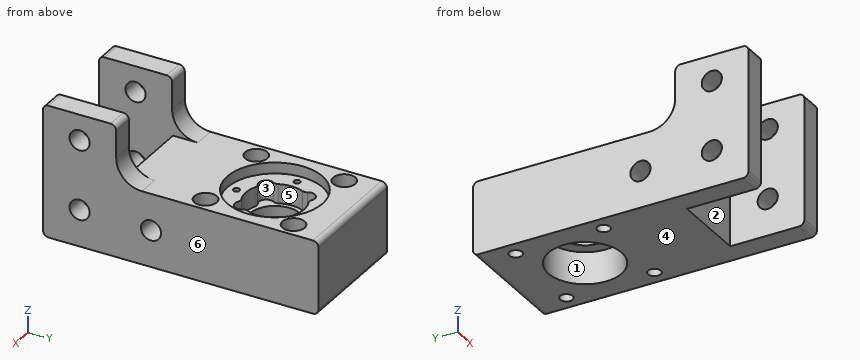
from build123d import *

# Parameters (mm, degrees)
EXTRUDE1_DEPTH      = 10.25
EXTRUDE1_DEPTH_BACK = 10.25
SKETCH1_W           = 20
SKETCH1_H           = 55
EXTRUDE2_DEPTH      = 6
SKETCH4_R           = 2.75
EXTRUDE3_DEPTH      = 78.393878957
SKETCH5_R           = 6.755
EXTRUDE4_DEPTH      = 77.273357078
FILLET2_R           = 1.5
SKETCH_1_W          = 32.5
SKETCH_1_H          = 73.75
CUT_EXTRUDE_1_DEPTH = 77.273357078
FILLET_1_R          = 1.5
SKETCH_2_R          = 13
CUT_EXTRUDE_2_DEPTH = 3
SKETCH_3_R          = 8
SKETCH_3_R_2        = 6.755
CUT_EXTRUDE_3_DEPTH = 5.25
FILLET_2_R          = 1.5
SKETCH_4_R          = 10
CUT_EXTRUDE_4_DEPTH = 8.75
SKETCH_5_R          = 0.875
CUT_EXTRUDE_5_DEPTH = 8
SKETCH_7_R          = 1.75
CUT_EXTRUDE_6_DEPTH = 71.154294238
SKETCH_8_R          = 3.05
CUT_EXTRUDE_7_DEPTH = 5


with BuildPart() as part:
    # Sketch1 → Extrude1 (new, two sides: drawn at the far end of the back side and taken through both)
    with BuildSketch(Plane(origin=(0, 0, 0), x_dir=(0, 0, -1), z_dir=(1, 0, 0)).offset(-EXTRUDE1_DEPTH_BACK)):
        with Locations((0, 37.75)):
            Rectangle(SKETCH1_W, SKETCH1_H)
    extrude(amount=EXTRUDE1_DEPTH + EXTRUDE1_DEPTH_BACK)

    # Sketch2 → Extrude2 (add)
    with BuildSketch(Plane(origin=(10.25, 0, 0), x_dir=(0, 0, -1), z_dir=(1, 0, 0))):
        with BuildLine():
            Line((26, 10), (17, 10))
            ThreePointArc((17, 10), (12.050252532, 12.050252532), (10, 17))
            Line((10, 17), (10, 65.25))
            Line((10, 65.25), (-10, 65.25))
            Line((-10, 65.25), (-10, 17))
            ThreePointArc((-10, 17), (-12.050252532, 12.050252532), (-17, 10))
            Line((-17, 10), (-26, 10))
            Line((-26, 10), (-26, -10))
            Line((-26, -10), (26, -10))
            Line((26, -10), (26, 10))
        make_face()
    extrude2 = extrude(amount=EXTRUDE2_DEPTH)

    # Mirror2: Extrude2 across plane
    add(extrude2.mirror(Plane(origin=(0, 0, 0), x_dir=(0, 0, 1), z_dir=(1, 0, 0))))

    # Sketch4 → Extrude3 (cut, through all)
    with BuildSketch(Plane(origin=(16.25, 0, 0), x_dir=(0, 0, -1), z_dir=(1, 0, 0))):
        Circle(SKETCH4_R)
        with Locations((19, 0)):
            Circle(SKETCH4_R)
        with Locations((-19, 0)):
            Circle(SKETCH4_R)
        with Locations((0, 19.5)):
            Circle(SKETCH4_R)
    extrude(amount=-EXTRUDE3_DEPTH, mode=Mode.SUBTRACT)

    # Sketch5 → Extrude4 (cut, through all)
    with BuildSketch(Plane.XY.offset(10)):
        with Locations((0, 44)):
            Circle(SKETCH5_R)
    extrude(amount=-EXTRUDE4_DEPTH, mode=Mode.SUBTRACT)

    # Fillet2
    fillet2_edges = [part.edges().sort_by_distance(p)[0] for p in [
        (13.25, 10, 26),
        (13.25, -10, 26),
        (13.25, -10, -26),
        (13.25, 10, -26),
        (-13.25, -10, 26),
        (-13.25, 10, 26),
        (-13.25, 10, -26),
        (-13.25, -10, -26),
        (0, 65.25, 10),
        (0, 65.25, -10),
    ]]
    fillet(fillet2_edges, radius=FILLET2_R)

    # Эскиз1 → Вырез-Вытянуть1 (cut, through all)
    with BuildSketch(Plane(origin=(0, 0, -10), x_dir=(-1, 0, 0), z_dir=(0, 0, -1))):
        with Locations((0, 26.875)):
            Rectangle(SKETCH_1_W, SKETCH_1_H)
    extrude(amount=CUT_EXTRUDE_1_DEPTH, mode=Mode.SUBTRACT)

    # Скругление1
    fillet_1_edges = [part.edges().sort_by_distance(p)[0] for p in [
        (-13.25, -10, -10),
        (13.25, -10, -10),
    ]]
    fillet(fillet_1_edges, radius=FILLET_1_R)

    # Эскиз2 → Вырез-Вытянуть2 (cut)
    with BuildSketch(Plane.XY.offset(10)):
        with Locations((0, 44)):
            Circle(SKETCH_2_R)
    extrude(amount=-CUT_EXTRUDE_2_DEPTH, mode=Mode.SUBTRACT)

    # Эскиз3 → Вырез-Вытянуть3 (cut)
    # profile 1 of 5: a face of its own
    with BuildSketch(Plane.XY.offset(7)):
        with Locations((0, 44)):
            Circle(SKETCH_3_R)
        with Locations((0, 44)):
            Circle(SKETCH_3_R_2, mode=Mode.SUBTRACT)
    # profile 2 of 5: a face of its own
    with BuildSketch(Plane.XY.offset(7)):
        with BuildLine():
            ThreePointArc((-6.883199074, 48.076956034), (-5.656854249, 49.656854249), (-4.076956034, 50.883199074))
            ThreePointArc((-4.076956034, 50.883199074), (-7.071067812, 51.071067812), (-6.883199074, 48.076956034))
        make_face()
    # profile 3 of 5: a face of its own
    with BuildSketch(Plane.XY.offset(7)):
        with BuildLine():
            ThreePointArc((4.076956034, 50.883199074), (5.656854249, 49.656854249), (6.883199074, 48.076956034))
            ThreePointArc((6.883199074, 48.076956034), (7.071067812, 51.071067812), (4.076956034, 50.883199074))
        make_face()
    # profile 4 of 5: a face of its own
    with BuildSketch(Plane.XY.offset(7)):
        with BuildLine():
            ThreePointArc((4.076956034, 37.116800926), (7.071067812, 36.928932188), (6.883199074, 39.923043966))
            ThreePointArc((6.883199074, 39.923043966), (5.656854249, 38.343145751), (4.076956034, 37.116800926))
        make_face()
    # profile 5 of 5: a face of its own
    with BuildSketch(Plane.XY.offset(7)):
        with BuildLine():
            ThreePointArc((-6.883199074, 39.923043966), (-7.071067812, 36.928932188), (-4.076956034, 37.116800926))
            ThreePointArc((-4.076956034, 37.116800926), (-5.656854249, 38.343145751), (-6.883199074, 39.923043966))
        make_face()
    extrude(amount=-CUT_EXTRUDE_3_DEPTH, mode=Mode.SUBTRACT)

    # Скругление2
    fillet_2_edges = [part.edges().sort_by_distance(p)[0] for p in [
        (6.883199074, 48.076956034, 4.375),
        (6.883199074, 39.923043966, 4.375),
        (4.076956034, 37.116800926, 4.375),
        (-4.076956034, 37.116800926, 4.375),
        (-6.883199074, 39.923043966, 4.375),
        (-6.883199074, 48.076956034, 4.375),
        (-4.076956034, 50.883199074, 4.375),
        (4.076956034, 50.883199074, 4.375),
    ]]
    fillet(fillet_2_edges, radius=FILLET_2_R)

    # Эскиз4 → Вырез-Вытянуть4 (cut)
    with BuildSketch(Plane(origin=(0, 0, -10), x_dir=(-1, 0, 0), z_dir=(0, 0, -1))):
        with Locations(Location((0, 44, 0), (0, 0, 90))):
            Circle(SKETCH_4_R)
    extrude(amount=-CUT_EXTRUDE_4_DEPTH, mode=Mode.SUBTRACT)

    # Эскиз5 → Вырез-Вытянуть5 (cut)
    with BuildSketch(Plane.XY.offset(7)):
        with Locations((0, 54.5)):
            Circle(SKETCH_5_R)
        with Locations((10.5, 44)):
            Circle(SKETCH_5_R)
        with Locations((0, 33.5)):
            Circle(SKETCH_5_R)
        with Locations((-10.5, 44)):
            Circle(SKETCH_5_R)
    extrude(amount=-CUT_EXTRUDE_5_DEPTH, mode=Mode.SUBTRACT)

    # Эскиз7 → Вырез-Вытянуть6 (cut, through all)
    with BuildSketch(Plane.XY.offset(10)):
        with Locations((-12.02081528, 56.02081528)):
            Circle(SKETCH_7_R)
        with Locations((12.02081528, 56.02081528)):
            Circle(SKETCH_7_R)
        with Locations((12.02081528, 31.97918472)):
            Circle(SKETCH_7_R)
        with Locations((-12.02081528, 31.97918472)):
            Circle(SKETCH_7_R)
    extrude(amount=-CUT_EXTRUDE_6_DEPTH, mode=Mode.SUBTRACT)

    # Эскиз8 → Вырез-Вытянуть7 (cut)
    with BuildSketch(Plane.XY.offset(10)):
        with Locations((-12.02081528, 56.02081528)):
            Circle(SKETCH_8_R)
        with Locations((12.02081528, 56.02081528)):
            Circle(SKETCH_8_R)
        with Locations((12.02081528, 31.97918472)):
            Circle(SKETCH_8_R)
        with Locations((-12.02081528, 31.97918472)):
            Circle(SKETCH_8_R)
    extrude(amount=-CUT_EXTRUDE_7_DEPTH, mode=Mode.SUBTRACT)


solid = part.part
Here's how the part is built. I have some questions about the finished solid (model axes, mm). Face numbers are marked on the shaded views. A direction names the side the tool comes from. Round coordinates to 2 decimals unless told otherwise and drop trailing zeros. Order: outer loops, then holes, each group sorted by start corner. A loop starts at its lowest first (then second) coordinate and runs counter-clockwise, first axis right, second up. Notation, with made-up numbers: M 72,27 L 82,27 A23 ccw 82,55 Z; hole C -27,82.25 d2. An arc over 180 degrees is marked long. One line per question, with ' | ' between items.
1) Imagine slicing it at A-A, the plane x = 0. Count the separate pieces of the cut face and the enclosed holes in it, plus the area to 3 significant figures.
Checked values:
separate pieces: 2 | enclosed holes: 1 | area: 670 mm²
2) Imagine slicing it at B-B, the plane y = 7.5. Write out the boundary of the cut face in (x, z).
Checked values:
outline: M -16.25,-10 L -10.25,-10 L -10.25,26 L -16.25,26 Z; M 10.25,-10 L 16.25,-10 L 16.25,26 L 10.25,26 Z
3) I need wall thicknesses on line 1 (X direction, y = 44, z = 4) (3 decimals); line 2 (X direction, y = -2, z = 15.5); line 3 (Y direction, x = -10.5, z = 1.5) (3 decimals). Which ranges of each line are inside material? Lowest first, please.
Checked values:
line 1: x = -16.25 to -11.375, -9.625 to -8, 8 to 9.625, 11.375 to 16.25 | line 2: x = -16.25 to -10.25, 10.25 to 16.25 | line 3: y = -10 to -2.305, 2.305 to 17.195, 21.805 to 31.113, 32.845 to 43.125, 44.875 to 55.155, 56.887 to 65.25
4) Imagine slicing it at C-C, the plane z = 19. Write out the boundary of the cut face in (x, y), plus the area to 3 significant figures.
Checked values:
outline: M -16.25,-10 L -10.25,-10 L -10.25,-2.75 L -16.25,-2.75 Z; M -16.25,2.75 L -10.25,2.75 L -10.25,10 L -16.25,10 Z; M 10.25,-10 L 16.25,-10 L 16.25,-2.75 L 10.25,-2.75 Z; M 10.25,2.75 L 16.25,2.75 L 16.25,10 L 10.25,10 Z | area: 174 mm²
5) We'd pull the mould along X, two halves only. Please class the marked faces 4, 5 and 6: released by +X, released by -X, zero draft, split by the parting line, or undercut.
Checked values:
face 4: zero draft | face 5: undercut | face 6: released by +X
6) On a 3-axis mill with a long thin cutter (end or side, diameter ignored), from which of +Z, -Z, +X, -X, +Y, -Y can I reach the whole of each face in a straight line? I mean the marked faces 1, 2 and 3. Say none if no direction works.
Checked values:
face 1: -Z | face 2: +Z, -Z, -Y | face 3: +Z
7) I'm going to push flat-ended pins straight in: pin 1 Ø2.5 at (x, y) = (0, 33.5) entering from +Z; pin 2 Ø15.5 at (x, y) = (0, 44) entering from -Z; pin 3 Ø3 at (x, y) = (-12.02, 31.98) entering from +Z; pin 4 Ø0.5 at (x, y) = (10.5, 43.5) entering from +Z. Where does each tip first touch, or does it pass through?
Checked values:
pin 1: stops at z = 7 | pin 2: stops at z = -1.25 | pin 3: passes through | pin 4: stops at z = -1
